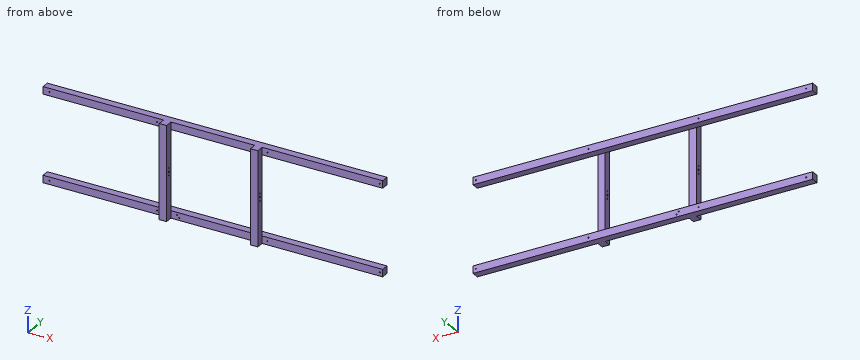
from build123d import *

# Parameters (mm, degrees)
ESBO_O1_W                  = 31.7
ESBO_O1_H                  = 405.7
RESSALTO_EXTRUS_O1_DEPTH   = 31.7
RESSALTO_EXTRUS_O1_2_DEPTH = 31.7
ESBO_O3_W                  = 1465.1
ESBO_O3_H                  = 31.7
RESSALTO_EXTRUS_O2_DEPTH   = 31.7
ESBO_O4_R                  = 2.5
CORTE_EXTRUS_O2_DEPTH      = 31.7
CORTE_EXTRUS_O3_DEPTH      = 761.777572619
CORTE_EXTRUS_O3_DEPTH_BACK = 761.777572619
ESBO_O5_R                  = 2.5
ESBO_O5_R_2                = 4


with BuildPart() as part:
    # Esbo_o1 → Ressalto-extrus_o1 (new body)
    with BuildSketch(Plane(origin=(0, 0, 0), x_dir=(1, 0, 0), z_dir=(0, 1, 0))):
        with Locations((-196.7, 0)):
            Rectangle(ESBO_O1_W, ESBO_O1_H)
    extrude(amount=-RESSALTO_EXTRUS_O1_DEPTH)



with BuildPart() as body_2:
    # Esbo_o1 → Ressalto-extrus_o1 2 (new body)
    with BuildSketch(Plane(origin=(0, 0, 0), x_dir=(1, 0, 0), z_dir=(0, 1, 0))):
        with Locations((196.7, 0)):
            Rectangle(ESBO_O1_W, ESBO_O1_H)
    extrude(amount=-RESSALTO_EXTRUS_O1_2_DEPTH)


with BuildPart() as part_1:
    add(part.part)

    add(body_2.part)  # Ressalto-extrus_o2 merges body 2
    # Esbo_o3 → Ressalto-extrus_o2 (add)
    with BuildSketch(Plane(origin=(0, 0, 0), x_dir=(1, 0, 0), z_dir=(0, 1, 0))):
        with Locations((0, 187)):
            Rectangle(ESBO_O3_W, ESBO_O3_H)
        with Locations((0, -187)):
            Rectangle(ESBO_O3_W, ESBO_O3_H)
    extrude(amount=RESSALTO_EXTRUS_O2_DEPTH)

    # Esbo_o4 → Corte-extrus_o2 (cut)
    with BuildSketch(Plane(origin=(0, 0, 0), x_dir=(1, 0, 0), z_dir=(0, 1, 0))):
        with Locations(Location((720, 187, 0), (0, 0, 270))):
            Circle(ESBO_O4_R)
        with Locations(Location((720, -187, 0), (0, 0, 270))):
            Circle(ESBO_O4_R)
        with Locations(Location((235.05, 187, 0), (0, 0, 270))):
            Circle(ESBO_O4_R)
        with Locations(Location((235.05, -187, 0), (0, 0, 270))):
            Circle(ESBO_O4_R)
        with Locations(Location((-704.55, 187, 0), (0, 0, 270))):
            Circle(ESBO_O4_R)
        with Locations(Location((-704.55, -187, 0), (0, 0, 270))):
            Circle(ESBO_O4_R)
        with Locations(Location((-240.55, 187, 0), (0, 0, 270))):
            Circle(ESBO_O4_R)
        with Locations(Location((-240.55, -187, 0), (0, 0, 270))):
            Circle(ESBO_O4_R)
        with Locations(Location((-155, 182, 0), (0, 0, 270))):
            Circle(ESBO_O4_R)
        with Locations(Location((-145, 192, 0), (0, 0, 270))):
            Circle(ESBO_O4_R)
    extrude(amount=CORTE_EXTRUS_O2_DEPTH, mode=Mode.SUBTRACT)

    # Esbo_o5 → Corte-extrus_o3 (cut, two sides: drawn at the far end of the back side and taken through both)
    with BuildSketch(Plane(origin=(0, 0, 0), x_dir=(0, 0, -1), z_dir=(1, 0, 0)).offset(-CORTE_EXTRUS_O3_DEPTH_BACK)):
        with Locations((16, -15.85)):
            Circle(ESBO_O5_R)
        with Locations((-16, -15.85)):
            Circle(ESBO_O5_R)
        with Locations((0, -15.85)):
            Circle(ESBO_O5_R_2)
    extrude(amount=CORTE_EXTRUS_O3_DEPTH + CORTE_EXTRUS_O3_DEPTH_BACK, mode=Mode.SUBTRACT)


solid = part_1.part
Check sheet for the modelled part. Datum: model origin and axes. Units: mm. Give positions to 0.01 mm unless a question says otherwise; leave off trailing zeros. Write each loop counter-clockwise with the first axis right and the second up, starting at its lowest first coordinate (ties: lowest second). Pieces come first, ordered by that corner, then holes. Notation, with made-up numbers: (-16.5, -38) -> (33.5, -38) arc R7 cw to (33.5, -33) -> close; hole circle Ø2 at (48, -35.75). An arc over 180 degrees is marked (long way). Write item = value, one per line.
Item 1: Sectioned sample at B-B on x = -3. Record the boundary of the cut face in (y, z), and give its area (3 significant figures).
Output:
outline = (0, -202.85) -> (31.7, -202.85) -> (31.7, -171.15) -> (0, -171.15) -> close; (0, 171.15) -> (31.7, 171.15) -> (31.7, 202.85) -> (0, 202.85) -> close
area = 2,010 mm^2
Item 2: Sectioned sample at A-A on y = 12. Count the separate pieces of the cut face and the enclosed holes in it, and give its area (3 significant figures).
Output:
separate_pieces = 2
enclosed_holes = 10
area = 92,700 mm^2
Item 3: Sectioned sample at C-C on z = 130. Record the boundary of the cut face in (x, y), and give its area (3 significant figures).
Output:
outline = (-212.55, -31.7) -> (-180.85, -31.7) -> (-180.85, 0) -> (-212.55, 0) -> close; (180.85, -31.7) -> (212.55, -31.7) -> (212.55, 0) -> (180.85, 0) -> close
area = 2,010 mm^2
Item 4: Scan lines: probe 1 along Z at (x, y) = (-155, 14); probe 2 along X at (y, z) = (24, 187); probe 3 along Z at (x, y) = (194, -15.85). Record each from-to range of solid material in increasing order. Write a range as from..to.
Output:
probe_1 = -202.85..-184.5, -179.5..-171.15, 171.15..202.85
probe_2 = -732.55..-707.05, -702.05..-243.05, -238.05..232.55, 237.55..717.5, 722.5..732.55
probe_3 = -202.85..-18.5, -13.5..-4, 4..13.5, 18.5..202.85
Item 5: Gauge pin test, flat ends, axial feed: pin 1 (8 mm diameter, centred on y = -15.85, z = 16, fed in from +X); pin 2 (6 mm diameter, centred on y = -25.5, z = -15.5, fed in from -X); pin 3 (6 mm diameter, centred on x = 720, z = -187, fed in from -Y). Record the tip position at first contact, or that the pin passes through.
Output:
pin_1 = 212.55
pin_2 = -212.55
pin_3 = 0
